Could you check a few things on this model? Use its own coordinates, in mm. Coordinates: 2 decimals unless noted, no trailing zeros. Loops run counter-clockwise (first coordinate to the right, second up) from the corner with the lowest first, then second, coordinate; pieces in that order, holes last.
from build123d import *

# Parameters (mm, degrees)
F1_DEPTH = 20
F2_D     = 10
F3_D     = 10
F0_W     = 120
F0_H     = 40
F0_W_2   = 40
F4_DEPTH = 20
F6_D     = 10


# Not quite as in the source:
# - a feature names something its author has since deleted; it is built from what else it names


with BuildPart() as f1:
    # F0 (on Top) → F1 (new body)
    with BuildSketch(Plane.XY):
        Polygon((-359.5256319247, 349.3264111251), (-559.5256319247, 349.3264111251), (-559.5256319247, -250.6735888749), (-359.5256319247, -250.6735888749), (-359.5256319247, -110.6735888749), (-359.5256319247, -70.6735888749), (-359.5256319247, 29.3264111251), (-399.5256319247, 29.3264111251), (-399.5256319247, -210.6735888749), (-519.5256319247, -210.6735888749), (-519.5256319247, 29.3264111251), (-519.5256319247, 69.3264111251), (-519.5256319247, 309.3264111251), (-399.5256319247, 309.3264111251), (-399.5256319247, 69.3264111251), (-359.5256319247, 69.3264111251), (-359.5256319247, 169.3264111251), (-359.5256319247, 209.3264111251), align=None)
    extrude(amount=F1_DEPTH)

    # F2 (through all)
    with Locations(Plane(origin=(0, 0, 0), x_dir=(1, 0, 0), z_dir=(0, 0, -1))):
        with Locations((-489.5256319247, -339.3264111251), (-429.5256319247, -319.3264111251), (-489.5256319247, -319.3264111251), (-489.5256319247, 220.6735888749), (-489.5256319247, 240.6735888749), (-429.5256319247, 240.6735888749), (-429.5256319247, 220.6735888749)):
            Hole(F2_D / 2)

    # F3 (through all)
    with Locations(Plane(origin=(0, 0, 0), x_dir=(1, 0, 0), z_dir=(0, 0, -1))):
        with Locations((-429.5256319247, -339.3264111251)):
            Hole(F3_D / 2)

    # F0 (on Top) → F4 (join)
    with BuildSketch(Plane.XY):
        with Locations((-459.5256319247, 49.3264111251)):
            Rectangle(F0_W, F0_H)
        with Locations((-379.5256319247, 49.3264111251)):
            Rectangle(F0_W_2, F0_H)
        Polygon((-109.5256319247, 29.3264111251), (-109.5256319247, 69.3264111251), (-188.0447282525, 69.3264111251), (-359.5256319247, 69.3264111251), (-359.5256319247, 29.3264111251), (-188.0447282525, 29.3264111251), align=None)
        Polygon((-109.5256319247, 69.3264111251), (-359.5256319247, 209.3264111251), (-359.5256319247, 169.3264111251), (-188.0447282525, 69.3264111251), align=None)
        Polygon((-359.5256319247, -70.6735888749), (-359.5256319247, -110.6735888749), (-109.5256319247, 29.3264111251), (-188.0447282525, 29.3264111251), align=None)
    extrude(amount=F4_DEPTH)

    # F6 (through all)
    with Locations(Plane.YZ.offset(-109.5256319247)):
        with Locations((49.3264111251, 10)):
            Hole(F6_D / 2)


solid = f1.part
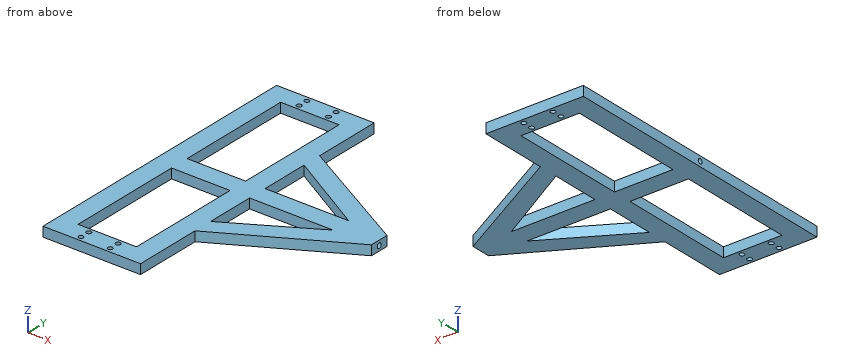
(1) I need wall thicknesses on probe 1 along Y at (x, z) = (-450.5, 10.5); probe 2 along Y at (x, z) = (-252, 10.25); probe 3 along X at (y, z) = (-202, 14.75). Which ranges of each line are inside material? Lowest first, please.
Answers:
probe 1: y = -250.67 to -210.67, 29.33 to 44.35, 54.3 to 69.33, 309.33 to 349.33
probe 2: y = -50.46 to -7.97, 29.33 to 44.33, 54.32 to 69.33, 106.62 to 149.11
probe 3: x = -559.53 to -519.53, -399.53 to -359.53
(2) Imagine slicing it at A-A, the plane x = -453. Write out the boundary of the cut face in (y, z).
Answers:
outline: (-250.67, 0) - (-210.67, 0) - (-210.67, 20) - (-250.67, 20) - close; (29.33, 0) - (69.33, 0) - (69.33, 20) - (29.33, 20) - close; (309.33, 0) - (349.33, 0) - (349.33, 20) - (309.33, 20) - close; hole circle Ø10 at (49.33, 10)
(3) Imagine slicing it at B-B, the plane z = 10. State how many separate pieces and enclosed holes the cut face has, and give its area (3 significant figures).
Answers:
separate pieces: 2
enclosed holes: 12
area: 85,100 mm2
(4) For pin 1 (9 mm diameter, centred on x = -429.53, y = 319.33, fed in from -Z); pin 2 (1.5 mm diameter, centred on x = -267.5, z = 9, fed in from -Y); pin 3 (6 mm diameter, centred on y = 125.5, z = 12.5, fed in from +X); pin 4 (10 mm diameter, centred on y = -12, z = 5.5, fed in from +X), each with a flat end and sliding along its axis, tell me the tip position at first contact or that it passes through.
Answers:
pin 1: passes through
pin 2: stops at y = -59.56
pin 3: stops at x = -204.48
pin 4: stops at x = -174.39
(5) Imagine slicing it at C-C, the plane y = -193. Write out the boundary of the cut face in (x, z).
Answers:
outline: (-559.53, 0) - (-519.53, 0) - (-519.53, 20) - (-559.53, 20) - close; (-399.53, 0) - (-359.53, 0) - (-359.53, 20) - (-399.53, 20) - close
(6) Imagine slicing it at D-D, the plane y = 134. Write out the boundary of the cut face in (x, z), and give its area (3 significant figures).
Answers:
outline: (-559.53, 0) - (-519.53, 0) - (-519.53, 20) - (-559.53, 20) - close; (-399.53, 0) - (-359.53, 0) - (-359.53, 20) - (-399.53, 20) - close; (-298.95, 0) - (-225.01, 0) - (-225.01, 20) - (-298.95, 20) - close
area: 3,080 mm2
